For this review, use the dimensioned drawing (mm, ordinates from the lowest corner) and the shaded views. A direction names the side the tool comes from. Round coordinates to 2 decimals unless told otherwise and drop trailing zeros. Order: outer loops, then holes, each group sorted by start corner. A loop starts at its lowest first (then second) coordinate and runs counter-clockwise, first axis right, second up. Notation, with made-up numbers: M 89.25,-34 L 124.25,-34 A26 cw 124.25,-1 Z; hole C -34.5,53 d9. An arc over 180 degrees is marked long. Use a Markdown table: item, result. Add a question column.
1. Consider section B-B on y = 17.25. Count the separate pieces of the cut face and the enclosed holes in it, then the cut area to 3 significant figures.
2. Insertion check: P1, Ø3, axis at y = 13, z = 12.5, coming from the +X side; P2, Ø5, axis at x = 4.5, z = 9, coming from the -Y side (1 decimal); P3, Ø6, axis at y = 12, z = 9.5, coming from the -X side. Each pin has a flat end and moves straight along its axis. Give the tip position at first contact, or say it passes through.
3. The part is to be moulded in two halves that separate along X. For the marked faces 3, 4 and 5, say which applies: +X half, -X half, draft (parallel to the pull), parting line (faces both ways), or undercut.
4. Consider section C-C on z = 13.5. State the section outline as (x, y) points (1 decimal).
5. Consider section A-A on z = 7.25. State the section outline as (x, y) points (1 decimal).
6. To check wall thickness, follow probe 1 along Z at (x, y) = (37, 20); probe 2 along X at (y, z) = (19, 7.5) (1 decimal); probe 3 along X at (y, z) = (14, 7) (1 decimal). State the ranges of each line that lie inside material, in increasing order.
7. For the marked faces 1 and 2, list the 3-axis set-ups (+Z, -Z, +X, -X, +Y, -Y) from which the entire face can be reached by the end or side of a thin tool; tool diameter is ignored.
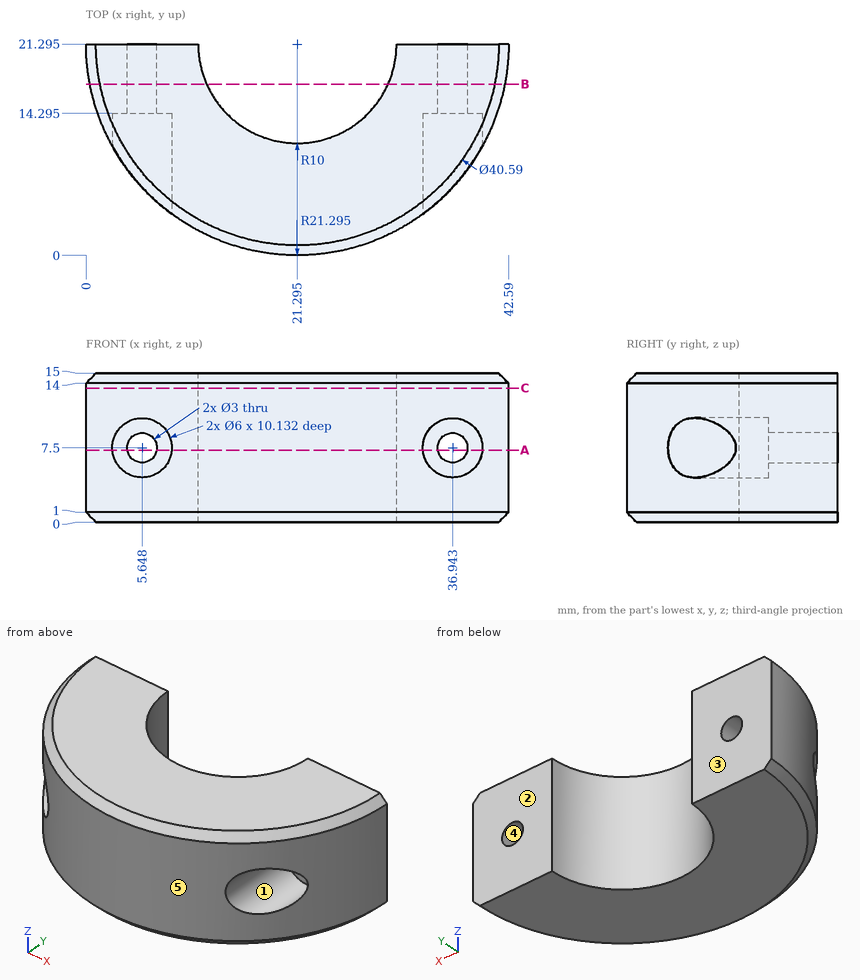
Answer block:
| question | item | result |
|---|---|---|
| 1 | separate pieces | 2 |
| 1 | enclosed holes | 2 |
| 1 | area | 337 mm^2 |
| 2 | P1 | x = 41.48 |
| 2 | P2 | y = 5.9 |
| 2 | P3 | x = 0.95 |
| 3 | face 3 | draft |
| 3 | face 4 | undercut |
| 3 | face 5 | parting line |
| 4 | outline | M 0,21.3 A21.3 ccw 42.6,21.3 L 31.3,21.3 A10 cw 11.3,21.3 Z |
| 5 | outline | M 0,21.3 A21.3 ccw 2.7,11 L 2.7,14.3 L 4.2,14.3 L 4.2,21.3 Z; M 7.1,14.3 L 8.6,14.3 L 8.6,4.2 A21.3 ccw 34,4.2 L 34,14.3 L 35.5,14.3 L 35.5,21.3 L 31.3,21.3 A10 cw 11.3,21.3 L 7.1,21.3 Z; M 38.4,14.3 L 39.9,14.3 L 39.9,11 A21.3 ccw 42.6,21.3 L 38.4,21.3 Z |
| 6 | probe 1 | 0 to 6, 9 to 15 |
| 6 | probe 2 | 0.1 to 4.1, 7.1 to 11.6, 31 to 35.4, 38.4 to 42.5 |
| 6 | probe 3 | 1.3 to 2.7, 8.6 to 14.5, 28.1 to 34, 39.9 to 41.3 |
| 7 | face 1 | -Y |
| 7 | face 2 | +Z, -Z, +X, -X, +Y |
